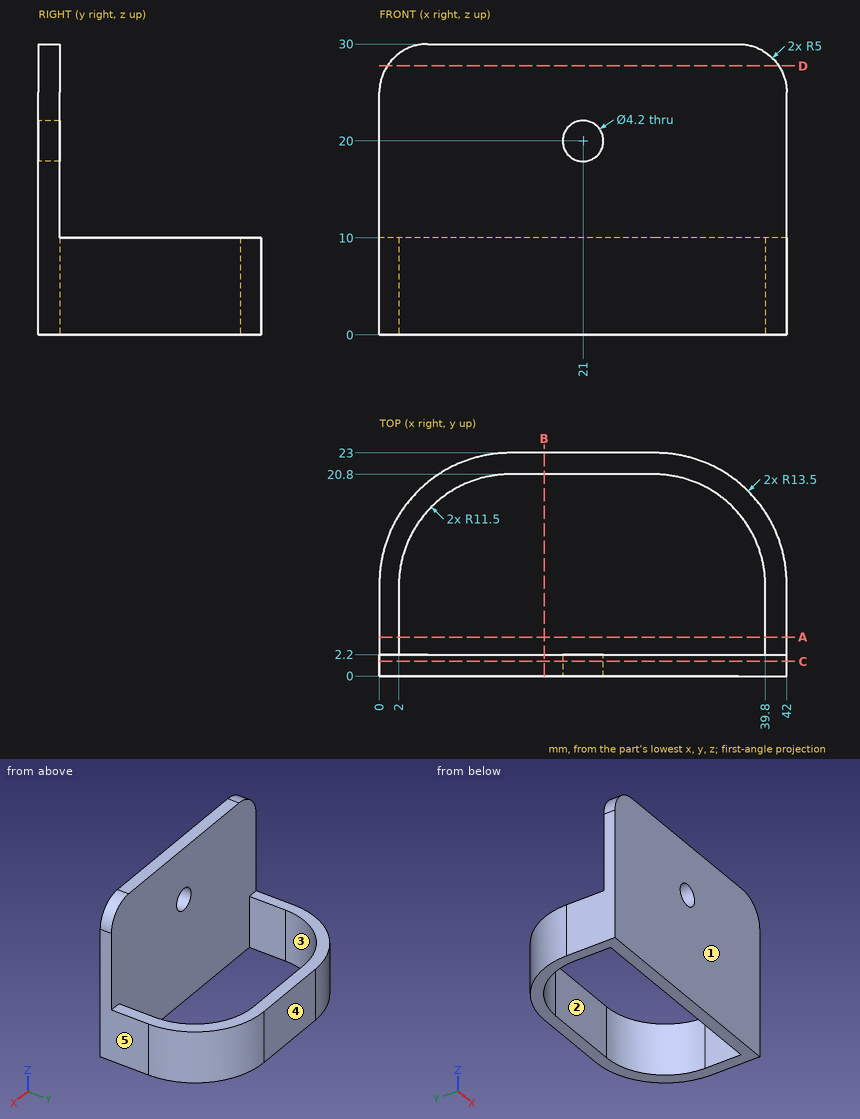
Here's the drawing with two shaded views (mm, measured from the low corner). I have some questions. A direction names the side the tool comes from. Coordinates: 2 decimals unless noted, no trailing zeros. Loops run counter-clockwise (first coordinate to the right, second up) from the corner with the lowest first, then second, coordinate; pieces in that order, holes last. Notation, with made-up numbers: (72.25, -24) -> (129.25, -24) arc R34 cw to (129.25, 13) -> close; hole circle Ø3 at (79.25, 77.5). An arc over 180 degrees is marked (long way). Answer as a JSON object with one key per item and string values.
1) Thinking about a two-plate mould opening in X: for the marked faces 3, 4 and 5, which applies, pulls with the +X half, pulls with the -X half, needs draft (parallel to the pull), parting line crosses it, or undercut?
Results:
{"face 3": "undercut", "face 4": "needs draft", "face 5": "pulls with the +X half"}
2) Imagine slicing it at A-A (y = 4). Please give me the cut outline in (x, z).
Results:
{"outline": "(0, 0) -> (2, 0) -> (2, 10) -> (0, 10) -> close; (39.8, 0) -> (42, 0) -> (42, 10) -> (39.8, 10) -> close"}
3) If I drill on line 1 (Z direction, x = 21, y = 1.15); line 2 (Y direction, x = 34, z = 23.5); line 3 (Y direction, x = 12, z = 1.75), over which ranges is the centre line in solid material (lowest first)?
Results:
{"line 1": "z = 0 to 17.9, 22.1 to 30", "line 2": "y = 0 to 2.2", "line 3": "y = 0 to 2.2, 20.7 to 22.92"}
4) For the marked faces 1 and 2, which set-ups out of +Z, -Z, +X, -X, +Y, -Y let a thin tool reach every point of the face, with its end or its side?
Results:
{"face 1": "+Z, -Z, +X, -X, -Y", "face 2": "+Z, -Z"}
5) Imagine slicing it at B-B (x = 17). Please give me the cut outline in (y, z), then the cut area to 3 significant figures.
Results:
{"outline": "(0, 0) -> (2.2, 0) -> (2.2, 30) -> (0, 30) -> close; (20.8, 0) -> (23, 0) -> (23, 10) -> (20.8, 10) -> close", "area": "88.0 mm^2"}
6) Imagine slicing it at C-C (y = 1.5). Please give me the cut outline in (x, z), then the cut area to 3 significant figures.
Results:
{"outline": "(0, 0) -> (42, 0) -> (42, 25) arc R5 ccw to (37, 30) -> (5, 30) arc R5 ccw to (0, 25) -> close; hole circle Ø4.2 at (21, 20)", "area": "1,240 mm^2"}
7) Imagine slicing it at D-D (z = 27.75). Please give me the cut outline in (x, y), then the cut area to 3 significant figures.
Results:
{"outline": "(0.82, 0) -> (41.18, 0) -> (41.18, 2.2) -> (0.82, 2.2) -> close", "area": "88.8 mm^2"}
8) For P1, Ø12, axis at x = 14, z = 24, coming from the +Y side; P2, Ø12, axis at y = 15.5, z = 12.5, coming from the +X side; P3, Ø10, axis at y = 20, z = 17.5, coming from the +X side, each with a flat end and sliding along its axis, tell me the tip position at first contact or that it passes through.
Results:
{"P1": "stops at y = 2.2", "P2": "stops at x = 41.99", "P3": "passes through"}
